from build123d import *

# Parameters (mm, degrees)
F0_W      = 100
F0_H      = 50
F1_DEPTH  = 100
F2_SIZE   = 5
F3_T      = -2
F4_W      = 80
F4_H      = 2
F5_DEPTH  = 50
F7_DEPTH  = 50
F8_W      = 2
F8_H      = 2
F9_DEPTH  = 4
F11_DEPTH = 50
F12_W     = 2
F12_H     = 2
F13_DEPTH = 4


with BuildPart() as f1:
    # F0 (on Front) → F1 (new body)
    with BuildSketch(Plane.XZ):
        with Locations((50, 25)):
            Rectangle(F0_W, F0_H)
    extrude(amount=F1_DEPTH)

    # F2
    f2_edges = [f1.edges().sort_by_distance(p)[0] for p in [
        (50, 0, 0),
        (0, -50, 0),
        (100, -50, 0),
        (0, -100, 25),
        (100, -100, 25),
        (100, 0, 25),
        (0, 0, 25),
    ]]
    chamfer(f2_edges, length=F2_SIZE)

    # F3
    f3_openings = [f1.faces().sort_by_distance(p)[0] for p in [
        (50, -50, 50),
    ]]
    offset(amount=F3_T, openings=f3_openings)

    # F4 (on face) → F5 (cut)
    with BuildSketch(Plane.XY.offset(50)):
        with Locations((50, -99)):
            Rectangle(F4_W, F4_H)
    extrude(amount=-F5_DEPTH, mode=Mode.SUBTRACT)

    # F6 (on face) → F7 (join)
    with BuildSketch(Plane(origin=(0, 0, 0), x_dir=(1, 0, 0), z_dir=(0, 0, -1))):
        Polygon((16, 102), (10, 102), (10, 100), (10, 98), (12, 98), (12, 100), (16, 100), align=None)
        Polygon((12, 98), (10, 98), (10, 96), (16, 96), (16, 98), align=None)
    extrude(amount=-F7_DEPTH)

    # F8 (on face) → F9 (join)
    with BuildSketch(Plane.YZ.offset(12)):
        with Locations((-99, 1)):
            Rectangle(F8_W, F8_H)
    extrude(amount=F9_DEPTH)

    # F10 (on face) → F11 (join)
    with BuildSketch(Plane(origin=(0, 0, 0), x_dir=(1, 0, 0), z_dir=(0, 0, -1))):
        Polygon((90, 100), (90, 102), (84, 102), (84, 100), (88, 100), (88, 98), (90, 98), align=None)
        Polygon((90, 96), (90, 98), (88, 98), (84, 98), (84, 96), align=None)
    extrude(amount=-F11_DEPTH)

    # F12 (on face) → F13 (join)
    with BuildSketch(Plane(origin=(88, 0, 0), x_dir=(0, -1, 0), z_dir=(-1, 0, 0))):
        with Locations((99, 1)):
            Rectangle(F12_W, F12_H)
    extrude(amount=F13_DEPTH)


solid = f1.part
Could you check a few things on this model? Use its own coordinates, in mm. A direction names the side the tool comes from. Give positions to 0.01 mm unless a question says otherwise; leave off trailing zeros. Loops run counter-clockwise (first coordinate to the right, second up) from the corner with the lowest first, then second, coordinate; pieces in that order, holes last. Notation, with made-up numbers: (18, 76.5) -> (27, 76.5) arc R25 cw to (27, 90.5) -> close; hole circle Ø6 at (59, -29.5). An arc over 180 degrees is marked (long way). Answer as CSV lines item,"result". Start each with the question number.
(1) If we section it at C-C on x = 85.5: Write out the boundary of the cut face in (y, z).
(2) I need wall thicknesses on probe 1 along X at (y, z) = (-39.5, 26); probe 2 along Z at (x, y) = (34.5, -42); probe 3 along Y at (x, z) = (63, 44.5). Which ranges of each line are inside material? Lowest first, please.
(3) If we section it at B-B on x = 73.5: Write out the boundary of the cut face in (y, z), then the cut area to 3 significant figures.
(4) If we section it at A-A on y = -78.5: Write out the boundary of the cut face in (x, z).
(5) I'm going to push flat-ended pins straight in: pin 1 Ø5 at (x, z) = (78.5, 7.5) entering from -Y; pin 2 Ø1.6 at (x, z) = (40, 1) entering from -Y; pin 3 Ø5 at (x, z) = (41, 43.5) entering from -Y. Where does each tip first touch, or does it pass through?
(6) Which directions (+Z, -Z, +X, -X, +Y, -Y) give clear straight access to the entire face, cutting with the end or side of a thin tool? Please do faces 1 (the flat face through (13, -102, 25)), 2 (the flat face through (95.679, -4.596, 4.548)), 3 (the flat face through (96.9, -3.5, 3.4)), 4 (the flat face through (7, -100, 25)), 5 (the flat face through (16, -101, 25)).
(7) We'd pull the mould along Y, two halves only. Please class faces 6 (the flat face through (87, -102, 25)), 7 (the flat face through (86, -100, 26)), 8 (the flat face through (1.6, -58.8, 50)): released by +Y, released by -Y, zero draft, split by the parting line, or undercut.
Computed:
1,outline,"(-102, 0) -> (-5, 0) -> (0, 5) -> (0, 50) -> (-2, 50) -> (-2, 5.83) -> (-5.83, 2) -> (-96, 2) -> (-96, 50) -> (-98, 50) -> (-98, 2) -> (-100, 2) -> (-100, 50) -> (-102, 50) -> close"
2,probe 1,"x = 0 to 2, 98 to 100"
2,probe 2,"z = 0 to 2"
2,probe 3,"y = -2 to 0"
3,outline,"(-98, 0) -> (-5, 0) -> (0, 5) -> (0, 50) -> (-2, 50) -> (-2, 5.83) -> (-5.83, 2) -> (-98, 2) -> close"
3,area,"287 mm2"
4,outline,"(0, 5) -> (5, 0) -> (95, 0) -> (100, 5) -> (100, 50) -> (98, 50) -> (98, 5.83) -> (94.17, 2) -> (5.83, 2) -> (2, 5.83) -> (2, 50) -> (0, 50) -> close"
5,pin 1,"stops at y = -2.83"
5,pin 2,"stops at y = -98"
5,pin 3,"stops at y = -2"
6,face 1,"+Z, -Z, +X, -X, -Y"
6,face 2,"+Z"
6,face 3,"-Z, +X, +Y"
6,face 4,"+Z, -Z, -X, -Y"
6,face 5,"+Z, -Z, -Y"
7,face 6,"released by -Y"
7,face 7,"undercut"
7,face 8,"zero draft"
